Autodesk Inventor part; units mm, degrees
ref_plane "YZ Plane" through (0, 0, 0) normal (1, 0, 0) x (0, 1, 0)
ref_plane "XZ Plane" through (0, 0, 0) normal (0, 1, 0) x (-1, 0, 0)
ref_plane "XY Plane" through (0, 0, 0) normal (0, 0, 1) x (1, 0, 0)
sketch "Sketch1" plane through (0, 0, 0) normal (0, 0, 1) x (1, 0, 0)
  line L0 (-7.8312, -44.5359) -> (133.0626, -44.5359)
  line L1 (133.0626, -44.5359) -> (133.0626, 47.9201)
  line L2 (133.0626, 47.9201) -> (-7.8312, 47.9201)
  line L3 (-7.8312, 47.9201) -> (-7.8312, -44.5359)
  line L4 (-7.8312, 47.9201) -> (-21.6516, 42.767)
  arc A0 (-21.6516, 42.767) -> (-23.7173, 39.7921) centre (-20.5423, 39.7921) ccw
  line L5 (-23.7173, 39.7921) -> (-23.7173, -36.4079)
  arc A1 (-23.7173, -36.4079) -> (-21.6516, -39.3828) centre (-20.5423, -36.4079) ccw
  line L6 (-21.6516, -39.3828) -> (-7.8312, -44.5359)
  circle A2 centre (-17.0085, 33.8104) radius 2.1971
  circle A3 centre (-17.0085, 27.689) radius 2.1971
  line L7 (-19.2056, 33.8104) -> (-14.8114, 33.8104)
  line L8 (-14.8114, 33.8104) -> (-14.8114, 27.689)
  line L9 (-14.8114, 27.689) -> (-19.2056, 27.689)
  line L10 (-19.2056, 27.689) -> (-19.2056, 33.8104)
  line L11 (-7.8312, 1.6921) -> (-23.7173, 1.6921)
  circle A4 centre (-17.0085, -30.4262) radius 2.1971
  circle A5 centre (-17.0085, -24.3048) radius 2.1971
  line L12 (-19.2056, -30.4262) -> (-14.8114, -30.4262)
  line L13 (-14.8114, -30.4262) -> (-14.8114, -24.3048)
  line L14 (-14.8114, -24.3048) -> (-19.2056, -24.3048)
  line L15 (-19.2056, -24.3048) -> (-19.2056, -30.4262)
  line L16 (62.6157, 47.9201) -> (62.6157, -44.5359)
  line L17 (133.0626, 47.9201) -> (146.8831, 42.767)
  arc A6 (148.9488, 39.7921) -> (146.8831, 42.767) centre (145.7738, 39.7921) ccw
  line L18 (148.9488, 39.7921) -> (148.9488, -36.4079)
  arc A7 (146.8831, -39.3828) -> (148.9488, -36.4079) centre (145.7738, -36.4079) ccw
  line L19 (146.8831, -39.3828) -> (133.0626, -44.5359)
  circle A8 centre (142.24, 33.8104) radius 2.1971
  circle A9 centre (142.24, 27.689) radius 2.1971
  line L20 (144.4371, 33.8104) -> (140.0429, 33.8104)
  line L21 (140.0429, 33.8104) -> (140.0429, 27.689)
  line L22 (140.0429, 27.689) -> (144.4371, 27.689)
  line L23 (144.4371, 27.689) -> (144.4371, 33.8104)
  line L24 (133.0626, 1.6921) -> (148.9488, 1.6921)
  circle A10 centre (142.24, -30.4262) radius 2.1971
  line L25 (144.4371, -30.4262) -> (140.0429, -30.4262)
  line L26 (140.0429, -30.4262) -> (140.0429, -24.3048)
  line L27 (140.0429, -24.3048) -> (144.4371, -24.3048)
  line L28 (144.4371, -24.3048) -> (144.4371, -30.4262)
  circle A11 centre (142.24, -24.3048) radius 2.1971
  point P0 (0, 0)
  point P1 (125.2315, 0)
  dimension "d4" = 4.3942
  dimension "d0" = 92.456
  dimension "d1" = 140.8938
  dimension "d2" = 3.175
  dimension "d3" = 76.2
  dimension "d5" = 6.1214
  dimension "d6" = 25.9969
extrude "Extrusion1" add sketch "Sketch1" along normal blind 3.175
sketch "Sketch2" plane through (0, 0, 3.175) normal (0, 0, 1) x (1, 0, 0)
  line L0 (133.0626, -44.5359) -> (-7.8312, -44.5359)
  line L1 (-7.8312, 47.9201) -> (133.0626, 47.9201)
  line L2 (7.1548, 47.9201) -> (118.0766, 47.9201)
  line L3 (121.2516, 44.7451) -> (121.2516, -41.3609)
  line L4 (118.0766, -44.5359) -> (7.1548, -44.5359)
  line L5 (3.9798, -41.3609) -> (3.9798, 44.7451)
  arc A0 (7.1548, 47.9201) -> (3.9798, 44.7451) centre (7.1548, 44.7451) ccw
  arc A1 (3.9798, -41.3609) -> (7.1548, -44.5359) centre (7.1548, -41.3609) ccw
  arc A2 (118.0766, -44.5359) -> (121.2516, -41.3609) centre (118.0766, -41.3609) ccw
  arc A3 (121.2516, 44.7451) -> (118.0766, 47.9201) centre (118.0766, 44.7451) ccw
  point P0 (0, 0)
  point P1 (3.9798, 47.9201)
  point P2 (121.2516, -44.5359)
  point P3 (62.6157, 47.9201)
  dimension "d9" = 117.2718
  dimension "d10" = 3.175
extrude "Extrusion2" add sketch "Sketch2" along normal blind 25.4
properties part number "LIDAR PSU"
Geometry check sheet. Reference: the model listing, model coordinates, mm. A direction names the side the tool comes from. Give positions to 0.01 mm unless a question says otherwise; leave off trailing zeros. Write each loop counter-clockwise with the first axis right and the second up, starting at its lowest first coordinate (ties: lowest second). Pieces come first, ordered by that corner, then holes.
1) Section check B-B, the plane x = 142.24. Record the boundary of the cut face in (y, z) (1 decimal).
2) Section check A-A, the plane z = 23.5. Record the boundary of the cut face in (x, y) (3 decimals).
3) Material ranges on L1, parallel to X at y = 37, z = 18.25; L2, parallel to Z at x = 142.5, y = 9 (3 decimals), recorded low to high.
4) Section check C-C, the plane y = -5. Record the boundary of the cut face in (x, z) (3 decimals).
5) Release check for a two-part mould opening along X. For faces 1 (the flat face through (144.437, -27, 2)), 2 (the flat face through (-14.838, -41.923, 1.565)), 3 (the flat face through (139.88, 45.38, 1.57)) record: pulls with the +X half, pulls with the -X half, needs draft (parallel to the pull), parting line crosses it, or undercut.
6) Gauge pin test, flat ends, axial feed: pin 1 (7.5 mm diameter, centred on y = -3.5, z = 20, fed in from +X); pin 2 (7.5 mm diameter, centred on y = -13.5, z = 13.5, fed in from -X); pin 3 (9.5 mm diameter, centred on x = -10, y = 1, fed in from +Z) (3 decimals); pin 4 (8 mm diameter, centred on x = 55, y = -26, fed in from -Z). Record the tip position at first contact, or that the pin passes through.
7) Section check D-D, the plane x = -2.5. Record the boundary of the cut face in (y, z) (3 decimals), and give its area (3 significant figures).
8) Access from +Z, -Z, +X, -X, +Y, -Y to the whole of each face (thin tool, end or side, straight path). Record for faces 4 (the cylindrical face through (4.935, -43.631, 15.697)), 5 (the flat face through (148.949, 2, 2)), 6 (the cylindrical face through (120.3, 47.01, 15.7)), 7 (the cylindrical face through (142.19, -22.11, 1.57)), 8 (the flat face through (121.252, 2, 16)).
Computed:
1. outline: (-41.1, 0) - (-32.6, 0) - (-32.6, 3.2) - (-41.1, 3.2) - close; (-22.1, 0) - (25.5, 0) - (25.5, 3.2) - (-22.1, 3.2) - close; (36, 0) - (44.5, 0) - (44.5, 3.2) - (36, 3.2) - close
2. outline: (3.98, -41.361) arc R3.175 ccw to (7.155, -44.536) - (118.077, -44.536) arc R3.175 ccw to (121.252, -41.361) - (121.252, 44.745) arc R3.175 ccw to (118.077, 47.92) - (7.155, 47.92) arc R3.175 ccw to (3.98, 44.745) - close
3. L1: x = 3.98 to 121.25
3. L2: z = 0 to 3.175
4. outline: (-23.717, 0) - (148.949, 0) - (148.949, 3.175) - (121.252, 3.175) - (121.252, 28.575) - (3.98, 28.575) - (3.98, 3.175) - (-23.717, 3.175) - close
5. face 1: undercut
5. face 2: pulls with the -X half
5. face 3: pulls with the +X half
6. pin 1: stops at x = 121.25
6. pin 2: stops at x = 3.98
6. pin 3: stops at z = 3.175
6. pin 4: stops at z = 0
7. outline: (-44.536, 0) - (47.92, 0) - (47.92, 3.175) - (-44.536, 3.175) - close
7. area: 294 mm2
8. face 4: +Z, -X, -Y
8. face 5: +Z, -Z, +X, +Y, -Y
8. face 6: +Z, +X, +Y
8. face 7: +Z, -Z
8. face 8: +Z, +X, +Y, -Y
